Could you check a few things on this model? Use its own coordinates, in mm. A direction names the side the tool comes from. Give positions to 0.01 mm unless a question says otherwise; leave off trailing zeros. Loops run counter-clockwise (first coordinate to the right, second up) from the corner with the lowest first, then second, coordinate; pieces in that order, holes last.
1. Imagine slicing it at B-B (x = -10.5). List the corners of the cut face in (y, z) for me (1 decimal).
2. For faces 1 (the flat face through (-37, -3.007, 29)), 2 (the flat face through (-37, -15.707, 36)), 3 (the flat face through (-37, -71.27, 20)), which set-ups out of +Z, -Z, +X, -X, +Y, -Y let a thin tool reach every point of the face, with its end or its side?
3. For P1, Ø4, axis at x = -66, z = 33.5, coming from the +Y side; P2, Ø16.5, axis at x = -8.93, y = 28.74, coming from the +Z side; P3, Ø4, axis at x = 9.5, y = 28.5, coming from the +Z side; P4, Ø3, axis at x = -35, y = -45, coming from the +Z side, each with a flat end and sliding along its axis, tell me the tip position at first contact or that it passes through.
4. I need wall thicknesses on line 1 along Z through (x, y) = (9, 29.5); line 2 along Y through (x, z) = (-66, 26); line 3 along Z through (x, y) = (-81.5, -55.5). Which ranges of each line are inside material? Lowest first, please.
5. Thinking about a two-plate mould opening in X: for faces 4 (the flat face through (22.821, -20, 16)), 5 (the cylindrical face through (-6.69, 18.67, 8.61)), 6 (the cylindrical face through (-72.436, 24.791, 8.609)), 7 (the flat face through (-37, 30, 17.462)), which applies, +X half, -X half, draft (parallel to the pull), parting line (faces both ways), or undercut?
6. Imagine slicing it at D-D (x = -25.5). List the corners of the cut face in (y, z) for me (1 decimal).
7. Imagine slicing it at A-A (z = 32.5). List the corners of the cut face in (x, y) for me.
8. Imagine slicing it at C-C (y = 26.5). List the corners of the cut face in (x, z) for me, plus the area to 3 significant figures.
```python
from build123d import *

# Parameters (mm, degrees)
F0_W     = 117.475
F0_H     = 133.35
F1_DEPTH = 17.4625
F3_D     = 20.6375
F2_W     = 117.475
F2_H     = 68.2625
F4_DEPTH = 12.7
F5_W     = 117.475
F5_H     = 12.7
F6_DEPTH = 11.1125


with BuildPart() as f1:
    # F0 (on Top) → F1 (new body)
    with BuildSketch(Plane.XY):
        with Locations((-35.916665, -4.594561)):
            Rectangle(F0_W, F0_H)
    extrude(amount=F1_DEPTH)

    # F3 (through all)
    with Locations(Plane.XY.offset(17.4625)):
        with Locations((-62.904165, 28.742939), (-8.929165, 28.742939)):
            Hole(F3_D / 2)

    # F2 (on face) → F4 (join)
    with BuildSketch(Plane.XY.offset(17.4625)):
        with Locations((-35.916665, -37.138311)):
            Rectangle(F2_W, F2_H)
    extrude(amount=F4_DEPTH)

    # F5 (on face) → F6 (join)
    with BuildSketch(Plane.XY.offset(30.1625)):
        with Locations((-35.916665, -9.357061)):
            Rectangle(F5_W, F5_H)
        Polygon((-94.654165, -71.269561), (22.820835, -71.269561), (22.820835, -59.890952), (-94.654165, -58.569561), align=None)
    extrude(amount=F6_DEPTH)


solid = f1.part
```
Derived:
1. outline: (-71.3, 0) - (18.5, 0) - (18.5, 17.5) - (-3, 17.5) - (-3, 41.3) - (-15.7, 41.3) - (-15.7, 30.2) - (-59.5, 30.2) - (-59.5, 41.3) - (-71.3, 41.3) - close; (38.9, 0) - (62.1, 0) - (62.1, 17.5) - (38.9, 17.5) - close
2. face 1: +Z, +X, -X, +Y
2. face 2: +Z, +X, -X
2. face 3: +Z, -Z, +X, -X, -Y
3. P1: stops at y = -3.01
3. P2: passes through
3. P3: stops at z = 17.46
3. P4: stops at z = 30.16
4. line 1: z = 0 to 17.46
4. line 2: y = -71.27 to -3.01
4. line 3: z = 0 to 30.16
5. face 4: +X half
5. face 5: undercut
5. face 6: undercut
5. face 7: draft
6. outline: (-71.3, 0) - (62.1, 0) - (62.1, 17.5) - (-3, 17.5) - (-3, 41.3) - (-15.7, 41.3) - (-15.7, 30.2) - (-59.3, 30.2) - (-59.3, 41.3) - (-71.3, 41.3) - close
7. outline: (-94.65, -71.27) - (22.82, -71.27) - (22.82, -59.89) - (-94.65, -58.57) - close; (-94.65, -15.71) - (22.82, -15.71) - (22.82, -3.01) - (-94.65, -3.01) - close
8. outline: (-94.65, 0) - (-72.98, 0) - (-72.98, 17.46) - (-94.65, 17.46) - close; (-52.83, 0) - (-19, 0) - (-19, 17.46) - (-52.83, 17.46) - close; (1.14, 0) - (22.82, 0) - (22.82, 17.46) - (1.14, 17.46) - close
8. area: 1,350 mm2
